from build123d import *

# Parameters (mm, degrees)
F1_W     = 60
F1_H     = 70
F2_DEPTH = 40
F3_T     = -2.5
F4_R     = 1.65
F4_R_2   = 2.5
F5_DEPTH = 20


with BuildPart() as f2:
    # F1 (on Top) → F2 (new body)
    with BuildSketch(Plane.XY):
        Rectangle(F1_W, F1_H)
    extrude(amount=F2_DEPTH)

    # F3
    f3_openings = [f2.faces().sort_by_distance(p)[0] for p in [
        (0, 0, 40),
    ]]
    offset(amount=F3_T, openings=f3_openings)

    # F4 (on face) → F5 (join)
    with BuildSketch(Plane.XY.offset(2.5)):
        with Locations((-23.15, -24.85)):
            Circle(F4_R)
        with Locations((19.85, 24.85)):
            Circle(F4_R)
        with Locations((20.5029603094, -26.5606511384)):
            Circle(F4_R)
        with Locations((-19.85, 24.85)):
            Circle(F4_R_2)
        with Locations((-19.85, 24.85)):
            Circle(F4_R, mode=Mode.SUBTRACT)
    extrude(amount=F5_DEPTH)


solid = f2.part
Design review of the part built by this model. Coordinates are the model's own, in mm. A direction names the side the tool comes from. Coordinates: 2 decimals unless noted, no trailing zeros. Write each loop counter-clockwise with the first axis right and the second up, starting at its lowest first coordinate (ties: lowest second). Pieces come first, ordered by that corner, then holes. Notation, with made-up numbers: (75.25, 12) -> (127.25, 12) arc R17 ccw to (127.25, 42) -> close; hole circle Ø6 at (44.25, -33). An arc over 180 degrees is marked (long way). Write each question's results on one line, items separated by ' | '. Start each with the question number.
(1) Take a section at A-A on z = 25. Write out the cut boundary in (x, y).
(2) Take a section at C-C on y = 24.85. Write out the cut boundary in (x, z), and give its area (4 significant figures).
(3) Tool access review of faces 4 (the face through (0, -35, 20)), 5 (the face through (-20, 25, 2.5)): name each direction out of +Z, -Z, +X, -X, +Y, -Y from which nothing blocks a thin tool from reaching the whole face with its end or side.
(4) Take a section at B-B on x = -10. Write out the cut boundary in (y, z), and give its area (4 significant figures).
(5) The part is to be moulded in two halves that separate along X. For faces 1 (the face through (-29, 0, 40)), 2 (the face through (19.49, 23.24, 12.36)), 3 (the face through (30, 0, 20)), say which applies: pulls with the +X half, pulls with the -X half, needs draft (parallel to the pull), parting line crosses it, or undercut.
(6) Take a section at D-D on z = 6. Write out the cut boundary in (x, y).
(7) Clearance check with flat-ended pins moving along their axes: P1, Ø8, axis at x = -21.5, y = -14.5, coming from the +Z side; P2, Ø4, axis at x = -21, y = 24.5, coming from the +Z side. State where each tip first meets the part, or that it passes through.
(8) For line 1 along X through (y, z) = (-12.5, 14); line 2 along Y through (x, z) = (-5.5, 15); line 3 along Y through (x, z) = (-19, 16), list the stretches that pass through material, from the lowest coordinate up. Write a range as from..to.
Results found:
1) outline: (-30, -35) -> (30, -35) -> (30, 35) -> (-30, 35) -> close; hole (-27.5, -32.5) -> (27.5, -32.5) -> (27.5, 32.5) -> (-27.5, 32.5) -> close
2) outline: (-30, 0) -> (30, 0) -> (30, 40) -> (27.5, 40) -> (27.5, 2.5) -> (21.5, 2.5) -> (21.5, 22.5) -> (18.2, 22.5) -> (18.2, 2.5) -> (-17.35, 2.5) -> (-17.35, 22.5) -> (-18.2, 22.5) -> (-18.2, 2.5) -> (-21.5, 2.5) -> (-21.5, 22.5) -> (-22.35, 22.5) -> (-22.35, 2.5) -> (-27.5, 2.5) -> (-27.5, 40) -> (-30, 40) -> close | area: 437.5 mm2
3) face 4: +Z, -Z, +X, -X, -Y | face 5: +Z
4) outline: (-35, 0) -> (35, 0) -> (35, 40) -> (32.5, 40) -> (32.5, 2.5) -> (-32.5, 2.5) -> (-32.5, 40) -> (-35, 40) -> close | area: 362.5 mm2
5) face 1: needs draft | face 2: undercut | face 3: pulls with the +X half
6) outline: (-30, -35) -> (30, -35) -> (30, 35) -> (-30, 35) -> close; circle Ø3.3 at (-23.15, -24.85); circle Ø5 at (-19.85, 24.85); circle Ø3.3 at (19.85, 24.85); circle Ø3.3 at (20.5, -26.56); hole (-27.5, -32.5) -> (27.5, -32.5) -> (27.5, 32.5) -> (-27.5, 32.5) -> close; hole circle Ø3.3 at (-19.85, 24.85)
7) P1: stops at z = 2.5 | P2: stops at z = 22.5
8) line 1: x = -30..-27.5, 27.5..30 | line 2: y = -35..-32.5, 32.5..35 | line 3: y = -35..-32.5, 22.5..23.44, 26.26..27.2, 32.5..35
